from build123d import *

# Parameters (mm, degrees)
F1_DEPTH = 25


with BuildPart() as f1:
    # F0 (on Top) → F1 (new body)
    with BuildSketch(Plane.XY):
        with BuildLine():
            Line((-68, -40.213773), (-68, -45.213773))
            Line((-68, -45.213773), (-38, -45.213773))
            Line((-38, -45.213773), (-38, -40.213773))
            Line((-38, -40.213773), (-28, -40.213773))
            Line((-28, -40.213773), (-28, -10.213773))
            Line((-28, -10.213773), (-32, -10.213773))
            Line((-32, -10.213773), (-32, -14.213773))
            ThreePointArc((-32, -14.213773), (-32.585786, -15.627986), (-34, -16.213773))
            Line((-34, -16.213773), (-38, -16.213773))
            ThreePointArc((-38, -16.213773), (-39.414214, -15.627986), (-40, -14.213773))
            Line((-40, -14.213773), (-40, -10.213773))
            Line((-40, -10.213773), (-48, -10.213773))
            Line((-48, -10.213773), (-48, -14.213773))
            ThreePointArc((-48, -14.213773), (-48.585786, -15.627986), (-50, -16.213773))
            Line((-50, -16.213773), (-54, -16.213773))
            ThreePointArc((-54, -16.213773), (-55.414214, -15.627986), (-56, -14.213773))
            Line((-56, -14.213773), (-56, -10.213773))
            Line((-56, -10.213773), (-64, -10.213773))
            Line((-64, -10.213773), (-88, -30.213773))
            Line((-88, -30.213773), (-88, -38.213773))
            ThreePointArc((-88, -38.213773), (-87.414214, -39.627986), (-86, -40.213773))
            Line((-86, -40.213773), (-68, -40.213773))
        make_face()
        with BuildLine():
            Line((-63, -26.213773), (-43, -26.213773))
            ThreePointArc((-43, -26.213773), (-39, -30.213773), (-43, -34.213773))
            Line((-43, -34.213773), (-63, -34.213773))
            ThreePointArc((-63, -34.213773), (-67, -30.213773), (-63, -26.213773))
        make_face(mode=Mode.SUBTRACT)
        with BuildLine():
            Line((-28, -10.213773), (-28, -40.213773))
            Line((-28, -40.213773), (-18, -40.213773))
            Line((-18, -40.213773), (-18, -45.213773))
            Line((-18, -45.213773), (12, -45.213773))
            Line((12, -45.213773), (12, -40.213773))
            Line((12, -40.213773), (30, -40.213773))
            ThreePointArc((30, -40.213773), (31.414214, -39.627986), (32, -38.213773))
            Line((32, -38.213773), (32, -30.213773))
            Line((32, -30.213773), (8, -10.213773))
            Line((8, -10.213773), (0, -10.213773))
            Line((0, -10.213773), (0, -14.213773))
            ThreePointArc((0, -14.213773), (-0.585786, -15.627986), (-2, -16.213773))
            Line((-2, -16.213773), (-6, -16.213773))
            ThreePointArc((-6, -16.213773), (-7.414214, -15.627986), (-8, -14.213773))
            Line((-8, -14.213773), (-8, -10.213773))
            Line((-8, -10.213773), (-16, -10.213773))
            Line((-16, -10.213773), (-16, -14.213773))
            ThreePointArc((-16, -14.213773), (-16.585786, -15.627986), (-18, -16.213773))
            Line((-18, -16.213773), (-22, -16.213773))
            ThreePointArc((-22, -16.213773), (-23.414214, -15.627986), (-24, -14.213773))
            Line((-24, -14.213773), (-24, -10.213773))
            Line((-24, -10.213773), (-28, -10.213773))
        make_face()
        with BuildLine():
            Line((7, -34.213773), (-13, -34.213773))
            ThreePointArc((-13, -34.213773), (-17, -30.213773), (-13, -26.213773))
            Line((-13, -26.213773), (7, -26.213773))
            ThreePointArc((7, -26.213773), (11, -30.213773), (7, -34.213773))
        make_face(mode=Mode.SUBTRACT)
    extrude(amount=F1_DEPTH)


solid = f1.part
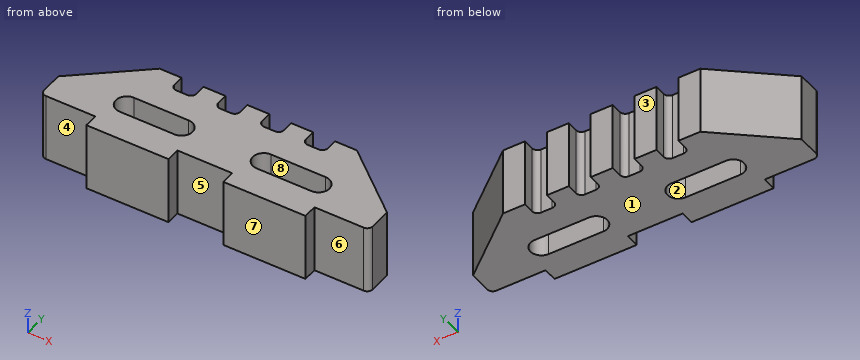
Can you work these out from the model? Positions are in its coordinate system, mm. Face numbers are marked on the shaded views. A direction names the side the tool comes from. Round coordinates to 2 decimals unless told otherwise and drop trailing zeros. Loops run counter-clockwise (first coordinate to the right, second up) from the corner with the lowest first, then second, coordinate; pieces in that order, holes last. Notation, with made-up numbers: (83, 73.5) - (113, 73.5) arc R11 ccw to (113, 77.5) - close; hole circle Ø2 at (74, 70.5). An arc over 180 degrees is marked (long way). Answer in a Markdown table with one row per item. Add a question column.
Q1. I need wall thicknesses on L1, parallel to X at y = -43, z = 9.5; L2, parallel to Y at x = -2, z = 19.5; L3, parallel to Y at x = -60.5, z = 5.75. Which ranges of each line are inside material? Lowest first, please.
Q2. For pin 1 Ø4 at (y, z) = (-43, 16) entering from -X; pin 2 Ø3 at (x, y) = (-20, -13.5) entering from +Z; pin 3 Ø1.2 at (y, z) = (-11.5, 18) entering from +X; pin 4 Ø4.5 at (y, z) = (-11.5, 11.5) entering from -X, each with a flat end and sliding along its axis, tell me the tip position at first contact or that it passes through.
Q3. I want a section at A-A on x = -52. List the corners of the cut face in (y, z) for me, and give its area (3 significant figures).
Q4. I want a section at D-D on x = -36. List the corners of the cut face in (y, z) for me.
Q5. I want a section at C-C on z = 6.25. Count the separate pieces of the cut face and the enclosed holes in it, and give its area (3 significant figures).
Q6. I want a section at B-B on x = 5.5. List the corners of the cut face in (y, z) for me, and give its area (3 significant figures).
Q7. We'd pull the mould along Y, two halves only. Please class the marked faces 1, 2 and 3: pulls with the +Y half, pulls with the -Y half, needs draft (parallel to the pull), parting line crosses it, or undercut.
Q8. Which directions (+Z, -Z, +X, -X, +Y, -Y) give clear straight access to the entire face, cutting with the end or side of a thin tool? Please do the marked faces 4, 5, 6, 7 and 8.
A:
| question | item | result |
|---|---|---|
| 1 | L1 | -68 to -38, -18 to 12 |
| 1 | L2 | -45.21 to -34.21, -26.21 to -16.21 |
| 1 | L3 | -45.21 to -34.21, -26.21 to -10.21 |
| 2 | pin 1 | x = -68 |
| 2 | pin 2 | through |
| 2 | pin 3 | x = 10.26 |
| 2 | pin 4 | x = -68.24 |
| 3 | outline | (-45.21, 0) - (-34.21, 0) - (-34.21, 25) - (-45.21, 25) - close; (-26.21, 0) - (-16.21, 0) - (-16.21, 25) - (-26.21, 25) - close |
| 3 | area | 525 mm^2 |
| 4 | outline | (-40.21, 0) - (-16.21, 0) - (-16.21, 25) - (-40.21, 25) - close |
| 5 | separate pieces | 1 |
| 5 | enclosed holes | 2 |
| 5 | area | 2,810 mm^2 |
| 6 | outline | (-45.21, 0) - (-34.21, 0) - (-34.21, 25) - (-45.21, 25) - close; (-26.21, 0) - (-10.21, 0) - (-10.21, 25) - (-26.21, 25) - close |
| 6 | area | 675 mm^2 |
| 7 | face 1 | needs draft |
| 7 | face 2 | undercut |
| 7 | face 3 | pulls with the +Y half |
| 8 | face 4 | +Z, -Z, -X, -Y |
| 8 | face 5 | +Z, -Z, -Y |
| 8 | face 6 | +Z, -Z, +X, -Y |
| 8 | face 7 | +Z, -Z, +X, -X, -Y |
| 8 | face 8 | +Z, -Z |
